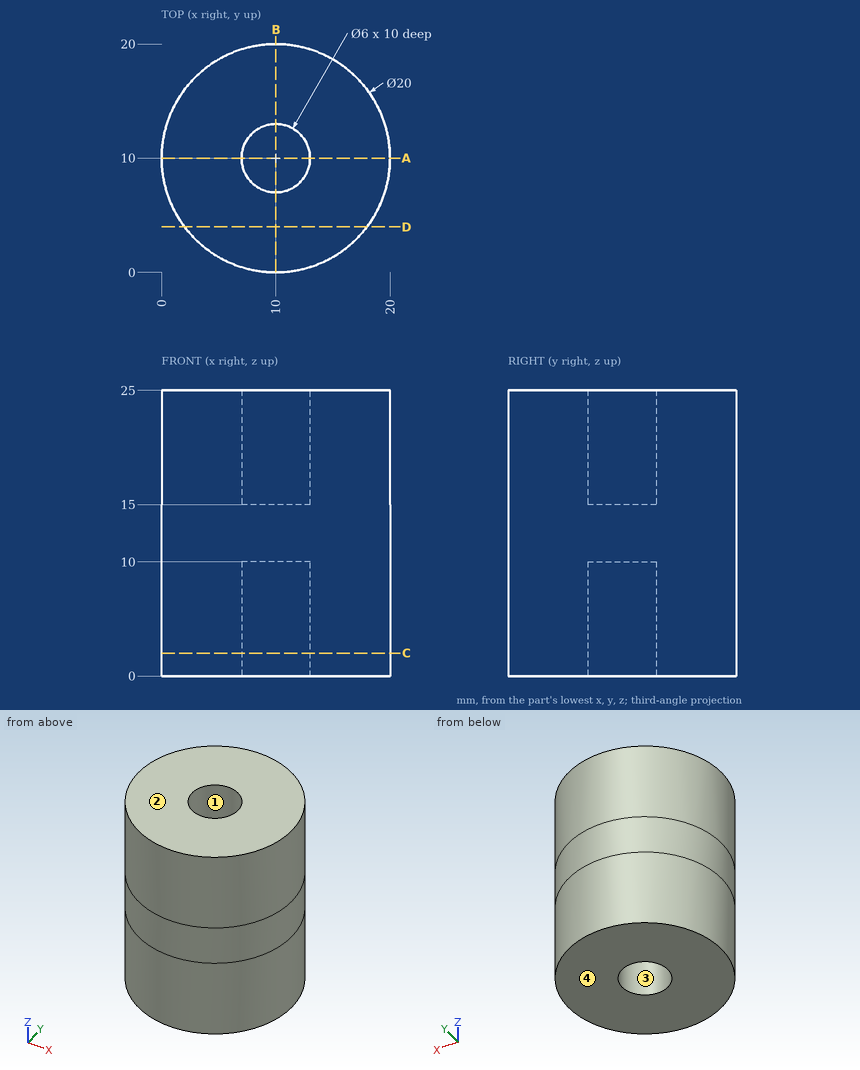
For this review, use the dimensioned drawing (mm, ordinates from the lowest corner) and the shaded views. A direction names the side the tool comes from. Round coordinates to 2 decimals unless told otherwise and drop trailing zeros. Order: outer loops, then holes, each group sorted by start corner. A loop starts at its lowest first (then second) coordinate and runs counter-clockwise, first axis right, second up.
1) Machinability: for the marked faces 3 and 4, which of the approach directions +Z, -Z, +X, -X, +Y, -Y give a long, thin tool a straight path to every point of the face, cutting with its end or side? Answer none if there is none.
The answers:
face 3: -Z
face 4: -Z, +X, -X, +Y, -Y
2) Clearance check with flat-ended pins moving along their axes: pin 1 Ø1.5 at (y, z) = (16, 15.5) entering from +X; pin 2 Ø2 at (y, z) = (7.5, 12.5) entering from -X; pin 3 Ø2 at (x, z) = (3, 13.5) entering from +Y. State where each tip first meets the part, or that it passes through.
The answers:
pin 1: stops at x = 18.51
pin 2: stops at x = 0.11
pin 3: stops at y = 18
3) Draft analysis for pull direction X (two halves, no side actions). For the marked faces 1 and 2, state which applies: released by +X, released by -X, zero draft, split by the parting line, or undercut.
The answers:
face 1: undercut
face 2: zero draft
4) Consider section C-C (z = 2). State the section outline as (x, y) points, plus the area to 3 significant figures.
The answers:
outline: circle Ø20 at (10, 10); hole circle Ø6 at (10, 10)
area: 286 mm2
5) Consider section A-A (y = 10). State the section outline as (x, z) points.
The answers:
outline: (0, 0) - (7, 0) - (7, 10) - (13, 10) - (13, 0) - (20, 0) - (20, 25) - (13, 25) - (13, 15) - (7, 15) - (7, 25) - (0, 25) - close
6) Consider section D-D (y = 4). State the section outline as (x, z) points, plus the area to 3 significant figures.
The answers:
outline: (2, 0) - (18, 0) - (18, 25) - (2, 25) - close
area: 400 mm2
7) For L1, parallel to Y at x = 10, z = 21.75; L2, parallel to Y at x = 11.75, z = 22.75; L3, parallel to Y at x = 1.5, z = 4.25, list the stretches that pass through material, from the lowest coordinate up.
The answers:
L1: y = 0 to 7, 13 to 20
L2: y = 0.15 to 7.56, 12.44 to 19.85
L3: y = 4.73 to 15.27
